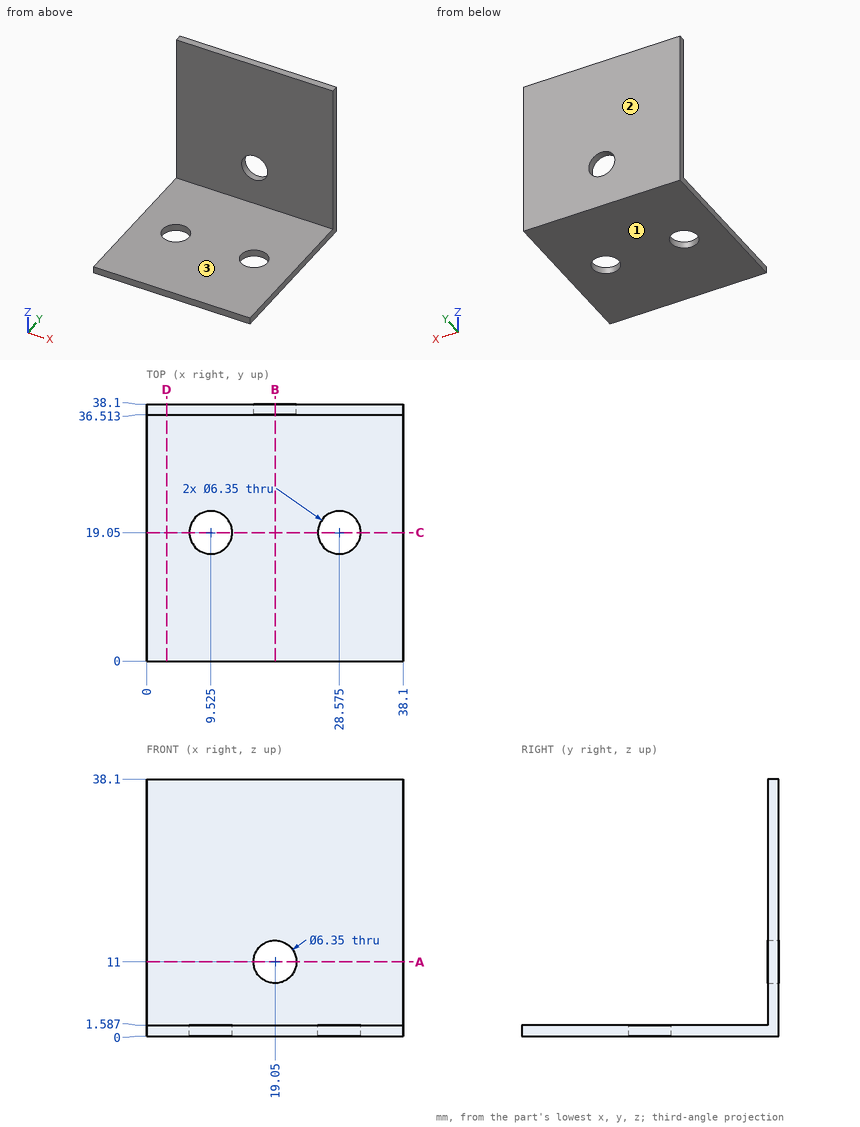
Job drawing, mm, ordinate dimensions from the low corner. One solid piece. Round coordinates to 2 decimals unless told otherwise and drop trailing zeros. Order: outer loops, then holes, each group sorted by start corner. A loop starts at its lowest first (then second) coordinate and runs counter-clockwise, first axis right, second up. Notation, with made-up numbers: (82, 81.25) - (96, 81.25) arc R11 ccw to (96, 91.25) - close; hole circle Ø4 at (42, 34). An arc over 180 degrees is marked (long way). Use CSV: the item, a comma, the result in double quotes. Start each with the question number.
1) Wall check: L1, parallel to X at y = 19.05, z = 0.8; L2, parallel to Z at x = 19.05, y = 36.8 (1 decimal); L3, parallel to Y at x = 26, z = 16. Give the ranges that are in metal, low to high. Write a range as [from, to].
2) Saw through at D-D (x = 3). List the corners of the cut face in (y, z).
3) Saw through at B-B (x = 19.05). List the corners of the cut face in (y, z) (1 decimal).
4) Pin check, flat tips, straight feed: pin 1 Ø6 at (x, z) = (23, 33) entering from -Y; pin 2 Ø11 at (x, y) = (25, 26.5) entering from +Z. Stop position of each tip, or through.
5) Saw through at A-A (z = 11). List the corners of the cut face in (x, y) (1 decimal).
6) Two-plate mould, pull along Z, no slides. Class the marked faces 1, 2 and 3: pulls with the +Z half, pulls with the -Z half, needs draft (parallel to the pull), parting line crosses it, or undercut.
7) Saw through at C-C (y = 19.05). List the corners of the cut face in (x, z).
Values follow:
1,L1,"x = [0, 6.35], [12.7, 25.4], [31.75, 38.1]"
1,L2,"z = [0, 7.8], [14.2, 38.1]"
1,L3,"y = [36.51, 38.1]"
2,outline,"(0, 0) - (38.1, 0) - (38.1, 38.1) - (36.51, 38.1) - (36.51, 1.59) - (0, 1.59) - close"
3,outline,"(0, 0) - (38.1, 0) - (38.1, 7.8) - (36.5, 7.8) - (36.5, 1.6) - (0, 1.6) - close; (36.5, 14.2) - (38.1, 14.2) - (38.1, 38.1) - (36.5, 38.1) - close"
4,pin 1,"stops at y = 36.51"
4,pin 2,"stops at z = 1.59"
5,outline,"(0, 36.5) - (15.9, 36.5) - (15.9, 38.1) - (0, 38.1) - close; (22.2, 36.5) - (38.1, 36.5) - (38.1, 38.1) - (22.2, 38.1) - close"
6,face 1,"pulls with the -Z half"
6,face 2,"needs draft"
6,face 3,"pulls with the +Z half"
7,outline,"(0, 0) - (6.35, 0) - (6.35, 1.59) - (0, 1.59) - close; (12.7, 0) - (25.4, 0) - (25.4, 1.59) - (12.7, 1.59) - close; (31.75, 0) - (38.1, 0) - (38.1, 1.59) - (31.75, 1.59) - close"
